The figure shows three views and two pictorial views of one solid part (mm, origin at its lowest corner). Answer the questions. A direction names the side the tool comes from. Round coordinates to 2 decimals unless told otherwise and drop trailing zeros. Write each loop counter-clockwise with the first axis right and the second up, starting at its lowest first coordinate (ties: lowest second). Pieces come first, ordered by that corner, then holes. Notation, with made-up numbers: (-17, 72.25) - (21, 72.25) arc R26 cw to (21, 87.25) - close; hole circle Ø11 at (77.25, -33.5). An arc over 180 degrees is marked (long way). Answer as CSV lines item,"result". Start each with the question number.
Item 1: A cutting plane is placed at C-C on y = 20. Determine the outline of the cut face in (x, z).
Item 2: A cutting plane is placed at A-A on y = 15. Determine the outline of the cut face in (x, z), and give its area (3 significant figures).
Item 3: Which of the six approach directions +Z, -Z, +X, -X, +Y, -Y give full straight-line access (tool end or side, diameter ignored) to the marked faces 1 and 2?
Item 4: Flat-ended cylindrical pins translate along their axes: pin 1 (10 mm diameter, centred on x = 47.5, z = 12.5, fed in from +Y); pin 2 (12.5 mm diameter, centred on x = 65.5, y = 14, fed in from -Z); pin 3 (2.5 mm diameter, centred on y = 2.5, z = 9, fed in from -X) (1 decimal). Find the tip coordinate at first contact, or state that the pin passes through.
Item 5: A cutting plane is placed at D-D on z = 19. Determine the outline of the cut face in (x, y) (1 decimal).
Item 6: Straight lines are drawn through the part: line 1 along X through (y, z) = (31, 53); line 2 along Y through (x, z) = (27, 19.5); line 3 along X through (y, z) = (4, 6.5) (1 decimal). For each, find the intervals that lie inside material, in ascending order. Write a range as [from, to].
Item 7: A cutting plane is placed at B-B on x = 24.25. Determine the outline of the cut face in (y, z), and give its area (3 significant figures).
Item 8: For a pull along X with two mould halves and no side action, classify the marked faces 3, 4, 5 and 6 as pulls with the +X half, pulls with the -X half, needs draft (parallel to the pull), parting line crosses it, or undercut.
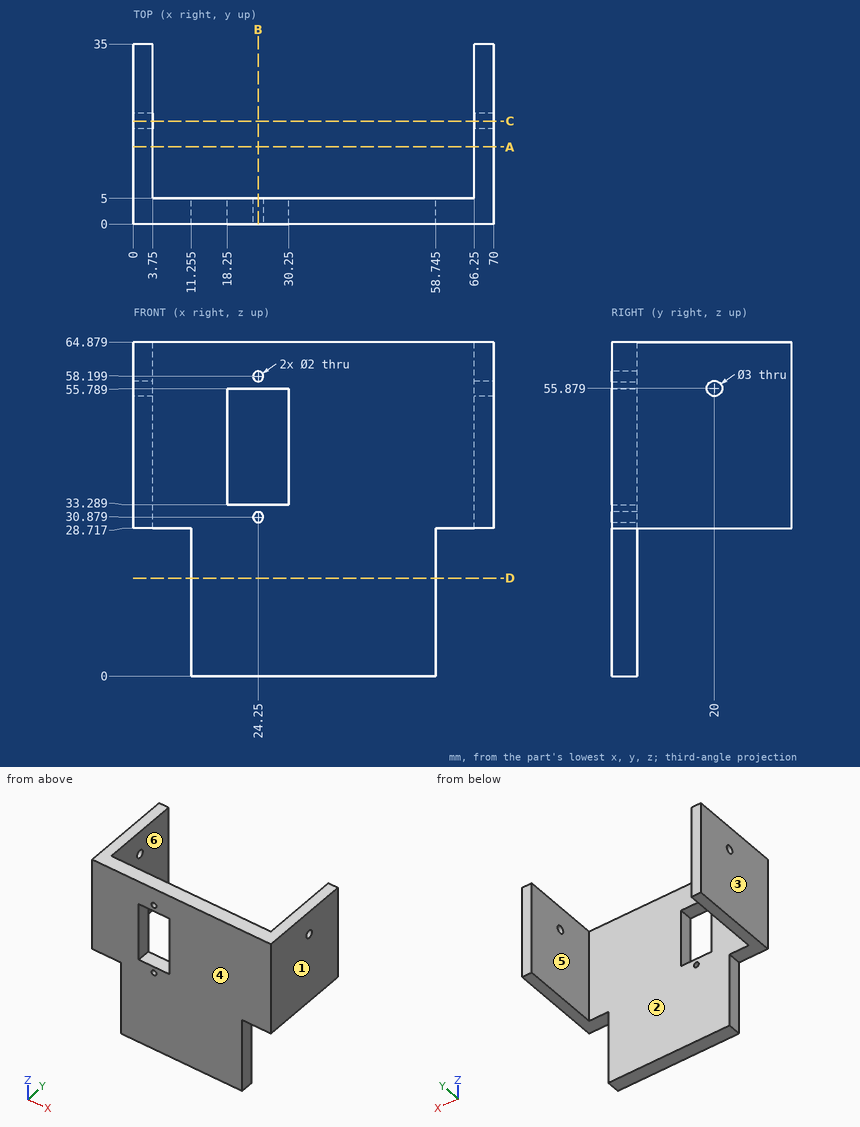
Geometry says:
1,outline,"(0, 28.72) - (3.75, 28.72) - (3.75, 54.38) - (0, 54.38) - close; (0, 57.38) - (3.75, 57.38) - (3.75, 64.88) - (0, 64.88) - close; (66.25, 28.72) - (70, 28.72) - (70, 54.38) - (66.25, 54.38) - close; (66.25, 57.38) - (70, 57.38) - (70, 64.88) - (66.25, 64.88) - close"
2,outline,"(0, 28.72) - (3.75, 28.72) - (3.75, 64.88) - (0, 64.88) - close; (66.25, 28.72) - (70, 28.72) - (70, 64.88) - (66.25, 64.88) - close"
2,area,"271 mm^2"
3,face 1,"+Z, -Z, +X, +Y, -Y"
3,face 2,"+Z, -Z, +Y"
4,pin 1,"stops at y = 5"
4,pin 2,"stops at z = 28.72"
4,pin 3,"stops at x = 11.3"
5,outline,"(11.3, 0) - (58.7, 0) - (58.7, 5) - (11.3, 5) - close"
6,line 1,"x = [0, 3.75], [66.25, 70]"
6,line 2,"y = [0, 5]"
6,line 3,"x = [11.3, 58.7]"
7,outline,"(0, 0) - (5, 0) - (5, 29.88) - (0, 29.88) - close; (0, 31.88) - (5, 31.88) - (5, 33.29) - (0, 33.29) - close; (0, 55.79) - (5, 55.79) - (5, 57.2) - (0, 57.2) - close; (0, 59.2) - (5, 59.2) - (5, 64.88) - (0, 64.88) - close"
7,area,"192 mm^2"
8,face 3,"pulls with the -X half"
8,face 4,"needs draft"
8,face 5,"undercut"
8,face 6,"undercut"
